Could you check a few things on this model? Use its own coordinates, in mm. Coordinates: 2 decimals unless noted, no trailing zeros. Loops run counter-clockwise (first coordinate to the right, second up) from the corner with the lowest first, then second, coordinate; pieces in that order, holes last. Notation, with made-up numbers: (70, 63) -> (112, 63) arc R14 cw to (112, 67) -> close; hole circle Ø11 at (46.25, -38.75). An arc over 180 degrees is marked (long way). One line per question, with ' | ' between items. Start each with the question number.
(1) I'm going to push flat-ended pins straight in: pin 1 Ø4 at (x, z) = (-28, 7) entering from +Y; pin 2 Ø2 at (x, z) = (29, 3.5) entering from +Y; pin 3 Ø4 at (y, z) = (21, 3) entering from -X. Where does each tip first touch, or does it pass through?
(2) Suppose I cut it at A-A (x = 0). Please give me the cut outline in (y, z) (3 decimals).
(3) Suppose I cut it at B-B (z = 1.25). Please give me the cut outline in (x, y) (3 decimals).
(4) If I drill on line 1 along Y through (x, z) = (0, 4); line 2 along Y through (x, z) = (-5.5, 5); line 3 along Y through (x, z) = (27, 4), over which ranges is the centre line in solid material (lowest first)?
```python
from build123d import *

# Parameters (mm, degrees)
F0_R     = 8.5
F1_DEPTH = 9.525
F2_R     = 2.54


# Not quite as in the source:
# - a feature names something its author has since deleted; it is built from what else it names


with BuildPart() as f1:
    # F0 (on Top) → F1 (new body)
    with BuildSketch(Plane.XY):
        with BuildLine():
            ThreePointArc((-12.1502250441, 23.4191023666), (-11.5002285841, 6.6396600688), (-26.3566501053, -1.1871476334))
            ThreePointArc((-26.3566501053, -1.1871476334), (-40.2545928187, -23.241), (-14.2064250612, -22.2319547331))
            ThreePointArc((-14.2064250612, -22.2319547331), (0, -13.2793201375), (14.2064250612, -22.2319547331))
            ThreePointArc((14.2064250612, -22.2319547331), (40.2545928187, -23.241), (26.3566501053, -1.1871476334))
            ThreePointArc((26.3566501053, -1.1871476334), (11.5002285841, 6.6396600688), (12.1502250441, 23.4191023666))
            ThreePointArc((12.1502250441, 23.4191023666), (0, 46.482), (-12.1502250441, 23.4191023666))
        make_face()
        with Locations((-27.4963065702, -15.875)):
            Circle(F0_R, mode=Mode.SUBTRACT)
        with Locations((27.4963065702, -15.875)):
            Circle(F0_R, mode=Mode.SUBTRACT)
        Circle(F0_R, mode=Mode.SUBTRACT)
        with Locations((0, 31.75)):
            Circle(F0_R, mode=Mode.SUBTRACT)
    extrude(amount=F1_DEPTH)

    # F2
    f2_edges = [f1.edges().sort_by_distance(p)[0] for p in [
        (-11.500229, 6.63966, 9.525),
    ]]
    fillet(f2_edges, radius=F2_R)


solid = f1.part
```
Checks:
1) pin 1: stops at y = -1.14 | pin 2: stops at y = -1.15 | pin 3: stops at x = -11.87
2) outline: (-13.279, 0) -> (-8.5, 0) -> (-8.5, 9.525) -> (-10.739, 9.525) arc R2.54 ccw to (-13.279, 6.985) -> close; (8.5, 0) -> (23.25, 0) -> (23.25, 9.525) -> (8.5, 9.525) -> close; (40.25, 0) -> (46.482, 0) -> (46.482, 6.985) arc R2.54 ccw to (43.942, 9.525) -> (40.25, 9.525) -> close
3) outline: (-26.357, -1.187) arc R14.732 ccw (long way) to (-14.206, -22.232) arc R15.748 cw to (14.206, -22.232) arc R14.732 ccw (long way) to (26.357, -1.187) arc R15.748 cw to (12.15, 23.419) arc R14.732 ccw (long way) to (-12.15, 23.419) arc R15.748 cw to start; hole circle Ø17 at (-27.496, -15.875); hole circle Ø17 at (0, 0); hole circle Ø17 at (0, 31.75); hole circle Ø17 at (27.496, -15.875)
4) line 1: y = -13.28 to -8.5, 8.5 to 23.25, 40.25 to 46.48 | line 2: y = -14.27 to -6.48, 6.48 to 25.27, 38.23 to 45.42 | line 3: y = -30.6 to -24.36, -7.39 to -1.15
